Geometry: final body of the model. Coordinates: model frame, mm. Round coordinates to 2 decimals unless told otherwise and drop trailing zeros. Write each loop counter-clockwise with the first axis right and the second up, starting at its lowest first coordinate (ties: lowest second). Pieces come first, ordered by that corner, then holes. Notation, with made-up numbers: M 56.5,-29 L 106.5,-29 A21 ccw 106.5,-9 Z; hole C -1.5,-18 d8. An arc over 180 degrees is marked long. Answer as CSV lines item,"result". Start each with the question number.
Q1. Section query A-A on z = 3.64. Output: boundary loops of the cut face in (x, y).
Q2. First-contact query: pin 1 (4.5 mm diameter, centred on x = 48.5, z = -11.5, fed in from -Y); pin 2 (4 mm diameter, centred on x = -48.5, z = -11.5, fed in from +Y). Flat tips, straight axial feed; report the tip coordinate or a pass-through.
Q3. Section query B-B on x = -36.85. Output: boundary loops of the cut face in (y, z).
Q4. Ray query, probe 1 along X at (y, z) = (-1, 4); probe 2 along X at (y, z) = (-0.1, 11.5); probe 3 along Z at (x, y) = (-36.85, -1.1). Return the intervals inside material, ascending.
Q5. Section query D-D on z = -11.5. Output: boundary loops of the cut face in (x, y).
Q6. Section query C-C on y = -0.7. Output: boundary loops of the cut face in (x, z), and give its area (3 significant figures).
Q7. Mould query, pull axis X, two halves, no side actions, for faces 1 (the cylindrical face through (51.4, -0.76, 14.45)), 2 (the cylindrical face through (32.856, -0.76, 3.926)), 3 (the cylindrical face through (-51.4, -0.76, 14.45)). Classes: pulls with the +X half, pulls with the -X half, needs draft (parallel to the pull), parting line crosses it, or undercut.
```python
from build123d import *

# Parameters (mm, degrees)
SKETCH_W            = 104.8
SKETCH_H            = 31
PAD_DEPTH           = 1.5
HOLE_D              = 3.4
HOLE_DEPTH          = 25
HOLE_CSINK_D        = 6.1
HOLE_CSINK_ANGLE    = 90
FILLET_R            = 3.5
SKETCH002_R         = 6.5
POCKET_DEPTH        = 1.501
LINEARPATTERN_COUNT = 2
LINEARPATTERN_PITCH = 76.2


with BuildPart() as part:
    # Sketch → Pad (new body)
    with BuildSketch(Plane.XZ):
        Rectangle(SKETCH_W, SKETCH_H)
    extrude(amount=PAD_DEPTH)

    # Hole
    with Locations(Plane.XZ.offset(1.5)):
        with Locations((-48.5, 11.5), (-48.5, -11.5), (48.5, -11.5), (48.5, 11.5)):
            CounterSinkHole(HOLE_D / 2, HOLE_CSINK_D / 2, depth=HOLE_DEPTH, counter_sink_angle=HOLE_CSINK_ANGLE)

    # Fillet
    fillet_edges = [part.edges().sort_by_distance(p)[0] for p in [
        (-52.4, -0.75, 15.5),
        (52.4, -0.75, 15.5),
    ]]
    fillet(fillet_edges, radius=FILLET_R)

    # Sketch002 (on Face5 of Fillet) → Pocket (cut, through all)
    with BuildSketch(Plane.XZ.offset(1.5)):
        with Locations((-36.85, 3.64)):
            Circle(SKETCH002_R)
    pocket = extrude(amount=-POCKET_DEPTH, mode=Mode.SUBTRACT)

    # LinearPattern: Pocket ×2
    with Locations(*[(i * LINEARPATTERN_PITCH, 0, 0) for i in range(1, LINEARPATTERN_COUNT)]):
        add(pocket, mode=Mode.SUBTRACT)


solid = part.part
```
Entries:
1,outline,"M -52.4,-1.5 L -43.35,-1.5 L -43.35,0 L -52.4,0 Z; M -30.35,-1.5 L 32.85,-1.5 L 32.85,0 L -30.35,0 Z; M 45.85,-1.5 L 52.4,-1.5 L 52.4,0 L 45.85,0 Z"
2,pin 1,"stops at y = -0.7"
2,pin 2,"stops at y = 0"
3,outline,"M -1.5,-15.5 L 0,-15.5 L 0,-2.86 L -1.5,-2.86 Z; M -1.5,10.14 L 0,10.14 L 0,15.5 L -1.5,15.5 Z"
4,probe 1,"x = -52.4 to -43.34, -30.36 to 32.86, 45.84 to 52.4"
4,probe 2,"x = -52.4 to -50.2, -46.8 to 46.8, 50.2 to 52.4"
4,probe 3,"z = -15.5 to -2.86, 10.14 to 15.5"
5,outline,"M -52.4,-1.5 L -51.55,-1.5 L -50.2,-0.15 L -50.2,0 L -52.4,0 Z; M -46.8,-0.15 L -45.45,-1.5 L 45.45,-1.5 L 46.8,-0.15 L 46.8,0 L -46.8,0 Z; M 50.2,-0.15 L 51.55,-1.5 L 52.4,-1.5 L 52.4,0 L 50.2,0 Z"
6,outline,"M -52.4,-15.5 L 52.4,-15.5 L 52.4,12 A3.5 ccw 48.9,15.5 L -48.9,15.5 A3.5 ccw -52.4,12 Z; hole C -48.5,-11.5 d4.5; hole C -48.5,11.5 d4.5; hole C -36.85,3.64 d13; hole C 39.35,3.64 d13; hole C 48.5,-11.5 d4.5; hole C 48.5,11.5 d4.5"
6,area,"2,910 mm^2"
7,face 1,"pulls with the +X half"
7,face 2,"undercut"
7,face 3,"pulls with the -X half"
